CAD build for the part. Positions are in the model's coordinates, mm. A direction names the side the tool comes from. Give positions to 0.01 mm unless a question says otherwise; leave off trailing zeros. Order: outer loops, then holes, each group sorted by start corner. A loop starts at its lowest first (then second) coordinate and runs counter-clockwise, first axis right, second up.
```python
from build123d import *

# Parameters (mm, degrees)
BOSS_EXTRUDE1_DEPTH = 6.35


with BuildPart() as part:
    # Sketch1 → Boss-Extrude1 (new body)
    with BuildSketch(Plane(origin=(0, 0, 0), x_dir=(1, 0, 0), z_dir=(0, 1, 0))):
        Polygon((-38.1, -38.1), (38.1, -38.1), (38.1, 38.1), (-38.1, 38.1), (-38.1, 24.13), (-46.2026, 24.13), (-46.2026, 20.447), (-44.0944, 20.447), (-44.0944, 17.78), (-51.9684, 17.78), (-51.9684, 20.447), (-49.8602, 20.447), (-49.8602, 24.13), (-57.9628, 24.13), (-57.9628, 9.9314), (-38.1, 9.9314), (-38.1, -9.9314), (-57.9628, -9.9314), (-57.9628, -24.13), (-49.8602, -24.13), (-49.8602, -20.447), (-51.9684, -20.447), (-51.9684, -17.78), (-44.0944, -17.78), (-44.0944, -20.447), (-46.2026, -20.447), (-46.2026, -24.13), (-38.1, -24.13), align=None)
        Polygon((-2.389310714, -18.580574179), (2.389310714, -18.580574179), (14.896593899, -11.359490865), (17.285904613, -7.221083314), (17.285904613, 7.221083314), (14.896593899, 11.359490865), (2.389310714, 18.580574179), (-2.389310714, 18.580574179), (-14.896593899, 11.359490865), (-17.285904613, 7.221083314), (-17.285904613, -7.221083314), (-14.896593899, -11.359490865), align=None, mode=Mode.SUBTRACT)
    extrude(amount=-BOSS_EXTRUDE1_DEPTH)


solid = part.part
```
Item 1: Drop flat-ended pins along their axis: pin 1 Ø3 at (y, z) = (-3.5, 32) entering from -X; pin 2 Ø1.9 at (x, y) = (-41.5, -4) entering from +Z; pin 3 Ø1.9 at (x, y) = (-52.5, -3) entering from -Z. Give the stop position or say it passes through.
Item 2: Two-plate mould, pull along X, no slides. Class faces 1 (the face through (-46.203, -3, 22)), 2 (the face through (-42, -3, 24.13)), 3 (the face through (-38.1, -3, 0)): released by +X, released by -X, zero draft, split by the parting line, or undercut.
Item 3: Slice it at B-B (x = 16). Give the cut face in (y, z), and give its area (3 significant figures).
Item 4: Slice it at A-A (z = 23). Give the cut face in (x, y), and give its area (3 significant figures).
Item 5: Tool access for faces 4 (the face through (-38.1, -3, -31)), 5 (the face through (-49.86, -3, -22)), 6 (the face through (-48, -3, 17.78)), 7 (the face through (-57.963, -3, 17)): list every direction of +Z, -Z, +X, -X, +Y, -Y with a clear straight run to the whole face (end or side of a thin tool).
Item 6: Wall check: L1, parallel to X at y = -6, z = -5.5; L2, parallel to X at y = -3.5, z = 18.5; L3, parallel to Z at x = 1, y = -5.5. Give the ranges that are in metal, low to high.
A:
1. pin 1: stops at x = -38.1
1. pin 2: stops at z = 24.13
1. pin 3: stops at z = -24.13
2. face 1: undercut
2. face 2: zero draft
2. face 3: released by -X
3. outline: (-6.35, -38.1) - (0, -38.1) - (0, -9.45) - (-6.35, -9.45) - close; (-6.35, 9.45) - (0, 9.45) - (0, 38.1) - (-6.35, 38.1) - close
3. area: 364 mm2
4. outline: (-57.96, -6.35) - (-49.86, -6.35) - (-49.86, 0) - (-57.96, 0) - close; (-46.2, -6.35) - (38.1, -6.35) - (38.1, 0) - (-46.2, 0) - close
4. area: 587 mm2
5. face 4: -Z, -X, +Y, -Y
5. face 5: -Z, +Y, -Y
5. face 6: +Y, -Y
5. face 7: +Z, -Z, -X, +Y, -Y
6. L1: x = -38.1 to -17.29, 17.29 to 38.1
6. L2: x = -57.96 to -51.97, -44.09 to -2.53, 2.53 to 38.1
6. L3: z = -38.1 to -18.58, 18.58 to 38.1
